from build123d import *

# Parameters (mm, degrees)
CYLINDER1840_R              = 74
CYLINDER1840_DEPTH          = 64
CYLINDER1831_R              = 2.5
CYLINDER1831_DEPTH          = 20
CYLINDER1830_R              = 2.5
CYLINDER1830_DEPTH          = 20
COMPOUND931_PLACEMENT_ANGLE = 90
CYLINDER1828_R              = 2.5
CYLINDER1828_DEPTH          = 20
CYLINDER1829_R              = 2.5
CYLINDER1829_DEPTH          = 20
COMPOUND930_PLACEMENT_ANGLE = 90
BOX785_W                    = 72
BOX785_H                    = 52
BOX785_DEPTH                = 6


with BuildPart() as obj1:
    # Cylinder1840 → Cylinder1840 (new body)
    with BuildSketch(Plane.XY.offset(25)):
        Circle(CYLINDER1840_R)
    extrude(amount=CYLINDER1840_DEPTH)


with BuildPart() as obj2:
    # Cylinder1831 → Cylinder1831 (new body)
    with BuildSketch(Plane(origin=(-90, -10, 66), x_dir=(1, 0, 0), z_dir=(0, 0, 1))):
        Circle(CYLINDER1831_R)
    extrude(amount=CYLINDER1831_DEPTH)


with BuildPart() as compound931:
    # Cylinder1830 → Cylinder1830 (new body)
    with BuildSketch(Plane(origin=(-110, -10, 66), x_dir=(1, 0, 0), z_dir=(0, 0, 1))):
        Circle(CYLINDER1830_R)
    extrude(amount=CYLINDER1830_DEPTH)

    # Compound931: union obj2
    add(obj2.part)


with BuildPart() as compound931_1:
    # Compound931 placement: moved
    add(compound931.part.moved(Location((-21.5, -8, 0))).rotate(Axis((-21.5, -8, 0), (0, 0, 1)), COMPOUND931_PLACEMENT_ANGLE))


with BuildPart() as obj3:
    # Cylinder1828 → Cylinder1828 (new body)
    with BuildSketch(Plane(origin=(-90, -10, 66), x_dir=(1, 0, 0), z_dir=(0, 0, 1))):
        Circle(CYLINDER1828_R)
    extrude(amount=CYLINDER1828_DEPTH)


with BuildPart() as compound932:
    # Cylinder1829 → Cylinder1829 (new body)
    with BuildSketch(Plane(origin=(-110, -10, 66), x_dir=(1, 0, 0), z_dir=(0, 0, 1))):
        Circle(CYLINDER1829_R)
    extrude(amount=CYLINDER1829_DEPTH)

    # Compound930: union obj3
    add(obj3.part)


with BuildPart() as compound932_1:
    # Compound930 placement: moved
    add(compound932.part.moved(Location((1.5, -8, 0))).rotate(Axis((1.5, -8, 0), (0, 0, 1)), COMPOUND930_PLACEMENT_ANGLE))

    # Compound932: union Compound931
    add(compound931_1.part)


with BuildPart() as cut597:
    # Box785 → Box785 (new body)
    with BuildSketch(Plane(origin=(26, -130, 78), x_dir=(0, 1, 0), z_dir=(0, 0, 1))):
        with Locations((36, 26)):
            Rectangle(BOX785_W, BOX785_H)
    extrude(amount=BOX785_DEPTH)

    # Cut594: cut Compound932
    add(compound932_1.part, mode=Mode.SUBTRACT)

    # Cut597: cut obj1
    add(obj1.part, mode=Mode.SUBTRACT)


solid = cut597.part
Geometry: final body of the model. Coordinates: model frame, mm. Coordinates: 2 decimals unless noted, no trailing zeros. Order: outer loops, then holes, each group sorted by start corner. A loop starts at its lowest first (then second) coordinate and runs counter-clockwise, first axis right, second up. Notation, with made-up numbers: M 39.5,-26 L 61.5,-26 A30 cw 61.5,8 Z; hole C 10,-15 d7. An arc over 180 degrees is marked long. One line per question, with ' | ' between items. Start each with the question number.
Item 1: Draft query along Y for faces 1 (the cylindrical face through (0, -74, 81)), 2 (the flat face through (0, -100, 78)), 3 (the flat face through (0, -130, 81)), 4 (the cylindrical face through (10.749, -115.615, 80.958)). Return one class per face: released by +Y, released by -Y, zero draft, split by the parting line, or undercut.
Item 2: Cut plane A-A, the plane y = -98. Return the cut outline in (x, z).
Item 3: Ray query, probe 1 along X at (y, z) = (-98, 80.6); probe 2 along X at (y, z) = (-119, 79.25); probe 3 along Y at (x, z) = (11.5, 79.65). Return the intervals inside material, ascending. Write a range as [from, to].
Item 4: Cut plane D-D, the plane x = -20.5. Return the cut outline in (y, z).
Item 5: Cut plane C-C, the plane z = 82.4. Return the cut outline in (x, y).
Item 6: Cut plane B-B, the plane x = 11.5. Return the cut outline in (y, z), then the cut area to 3 significant figures.
Item 7: Pin query (flat end, axial travel): pin 1 Ø4.5 at (x, y) = (-11.5, -98) entering from -Z; pin 2 Ø1 at (x, z) = (-8, 80) entering from +Y; pin 3 Ø1 at (x, z) = (0, 80.5) entering from +Y. Return the tip coordinate at first contact, or that it passes through.
A:
1) face 1: released by +Y | face 2: zero draft | face 3: released by -Y | face 4: undercut
2) outline: M -26,78 L -14,78 L -14,84 L -26,84 Z; M -9,78 L 9,78 L 9,84 L -9,84 Z; M 14,78 L 26,78 L 26,84 L 14,84 Z
3) probe 1: x = [-26, -14], [-9, 9], [14, 26] | probe 2: x = [-26, -13.79], [-9.21, 9.21], [13.79, 26] | probe 3: y = [-130, -120.5], [-115.5, -100.5], [-95.5, -73.1]
4) outline: M -130,78 L -71.1,78 L -71.1,84 L -130,84 Z
5) outline: M -26,-130 L 26,-130 L 26,-69.28 A74 cw -26,-69.28 Z; hole C -11.5,-118 d5; hole C -11.5,-98 d5; hole C 11.5,-118 d5; hole C 11.5,-98 d5
6) outline: M -130,78 L -120.5,78 L -120.5,84 L -130,84 Z; M -115.5,78 L -100.5,78 L -100.5,84 L -115.5,84 Z; M -95.5,78 L -73.1,78 L -73.1,84 L -95.5,84 Z | area: 281 mm2
7) pin 1: passes through | pin 2: stops at y = -73.51 | pin 3: stops at y = -74
